Part model, mm, in its own coordinate system. A direction names the side the tool comes from. Round coordinates to 2 decimals unless told otherwise and drop trailing zeros. Order: outer loops, then holes, each group sorted by start corner. A loop starts at its lowest first (then second) coordinate and runs counter-clockwise, first axis right, second up. Notation, with made-up numbers: (12, 87.5) - (44, 87.5) arc R15 ccw to (44, 94.5) - close; hole circle Ø8 at (21.25, 5). An arc over 180 degrees is marked (long way). Return JSON: item names as keys, results as strings. Group by question number.
Item 1: Probe probe 1 along Y at (x, z) = (-27.5, 2.85); probe 2 along X at (y, z) = (-1.5, 2.2); probe 3 along X at (y, z) = (-0.5, 1.25). List the from-to ranges inside material, lowest first.
Item 2: Drop flat-ended pins along their axis: pin 1 (1 mm diameter, centred on y = 0.5, z = 4, fed in from -X); pin 2 (4 mm diameter, centred on x = 61.5, y = 1, fed in from +Z). Give the stop position or say it passes through.
Item 3: Saw through at B-B on z = 1.35. List the corners of the cut face in (x, y) (3 decimals).
Item 4: Two-plate mould, pull along X, no slides. Class faces 1 (the face through (-1, 1.651, 3)), 2 (the face through (-53.086, -0.036, 2.504)), 3 (the face through (55.625, -0.092, 3.792)), 4 (the face through (1, 4.191, 3)): released by +X, released by -X, zero draft, split by the parting line, or undercut.
Item 5: Tool access for faces 5 (the face through (-1, -4.191, 3)), 6 (the face through (-55.625, 0.092, 3.792)), 7 (the face through (1, -1.651, 3)): list every direction of +Z, -Z, +X, -X, +Y, -Y with a clear straight run to the whole face (end or side of a thin tool).
Item 6: Saw through at C-C on y = 0. List the corners of the cut face in (x, z).
Item 7: Saw through at A-A on x = -48. List the corners of the cut face in (y, z).
```python
from build123d import *

# Parameters (mm, degrees)
F1_DEPTH = 2.54
F3_DEPTH = 2.54


with BuildPart() as f1:
    # F0 (on Top) → F1 (new body)
    with BuildSketch(Plane.XY):
        with BuildLine():
            Line((76.835, 4.191), (-76.835, 4.191))
            ThreePointArc((-76.835, 4.191), (-81.026, 0), (-76.835, -4.191))
            Line((-76.835, -4.191), (76.835, -4.191))
            ThreePointArc((76.835, -4.191), (81.026, 0), (76.835, 4.191))
        make_face()
        with BuildLine():
            ThreePointArc((-76.835, -1.651), (-78.486, 0), (-76.835, 1.651))
            Line((-76.835, 1.651), (-64.135, 1.651))
            ThreePointArc((-64.135, 1.651), (-62.484, 0), (-64.135, -1.651))
            Line((-64.135, -1.651), (-76.835, -1.651))
        make_face(mode=Mode.SUBTRACT)
        with BuildLine():
            Line((51.435, -1.651), (-51.435, -1.651))
            ThreePointArc((-51.435, -1.651), (-53.086, 0), (-51.435, 1.651))
            Line((-51.435, 1.651), (51.435, 1.651))
            ThreePointArc((51.435, 1.651), (53.086, 0), (51.435, -1.651))
        make_face(mode=Mode.SUBTRACT)
        with BuildLine():
            ThreePointArc((76.835, 1.651), (78.486, 0), (76.835, -1.651))
            Line((76.835, -1.651), (64.135, -1.651))
            ThreePointArc((64.135, -1.651), (62.484, 0), (64.135, 1.651))
            Line((64.135, 1.651), (76.835, 1.651))
        make_face(mode=Mode.SUBTRACT)
    extrude(amount=F1_DEPTH)

    # F2 (on face) → F3 (join)
    with BuildSketch(Plane.XY.offset(2.54)):
        with BuildLine():
            Line((51.435, 4.191), (-51.435, 4.191))
            ThreePointArc((-51.435, 4.191), (-55.626, 0), (-51.435, -4.191))
            Line((-51.435, -4.191), (51.435, -4.191))
            ThreePointArc((51.435, -4.191), (55.626, 0), (51.435, 4.191))
        make_face()
        with BuildLine():
            ThreePointArc((-51.435, -1.651), (-53.086, 0), (-51.435, 1.651))
            Line((-51.435, 1.651), (51.435, 1.651))
            ThreePointArc((51.435, 1.651), (53.086, 0), (51.435, -1.651))
            Line((51.435, -1.651), (-51.435, -1.651))
        make_face(mode=Mode.SUBTRACT)
    extrude(amount=F3_DEPTH)


solid = f1.part
```
Filled in:
{
 "1": {"probe 1": "y = -4.19 to -1.65, 1.65 to 4.19", "probe 2": "x = -80.75 to -77.52, -63.45 to -52.12, 52.12 to 63.45, 77.52 to 80.75", "probe 3": "x = -81 to -78.41, -62.56 to -53.01, 53.01 to 62.56, 78.41 to 81"},
 "2": {"pin 1": "stops at x = -55.63", "pin 2": "stops at z = 2.54"},
 "3": {"outline": "(-76.835, -4.191) - (76.835, -4.191) arc R4.191 ccw to (76.835, 4.191) - (-76.835, 4.191) arc R4.191 ccw to start; hole (-76.835, -1.651) - (-64.135, -1.651) arc R1.651 ccw to (-64.135, 1.651) - (-76.835, 1.651) arc R1.651 ccw to start; hole (-51.435, -1.651) - (51.435, -1.651) arc R1.651 ccw to (51.435, 1.651) - (-51.435, 1.651) arc R1.651 ccw to start; hole (64.135, -1.651) - (76.835, -1.651) arc R1.651 ccw to (76.835, 1.651) - (64.135, 1.651) arc R1.651 ccw to start"},
 "4": {"face 1": "undercut", "face 2": "undercut", "face 3": "released by +X", "face 4": "zero draft"},
 "5": {"face 5": "+Z, -Z, +X, -X, -Y", "face 6": "+Z, -X", "face 7": "+Z, -Z"},
 "6": {"outline": "(-81.03, 0) - (-78.49, 0) - (-78.49, 2.54) - (-81.03, 2.54) - close; (-62.48, 0) - (-53.09, 0) - (-53.09, 5.08) - (-55.63, 5.08) - (-55.63, 2.54) - (-62.48, 2.54) - close; (53.09, 0) - (62.48, 0) - (62.48, 2.54) - (55.63, 2.54) - (55.63, 5.08) - (53.09, 5.08) - close; (78.49, 0) - (81.03, 0) - (81.03, 2.54) - (78.49, 2.54) - close"},
 "7": {"outline": "(-4.19, 0) - (-1.65, 0) - (-1.65, 5.08) - (-4.19, 5.08) - close; (1.65, 0) - (4.19, 0) - (4.19, 5.08) - (1.65, 5.08) - close"}
}
